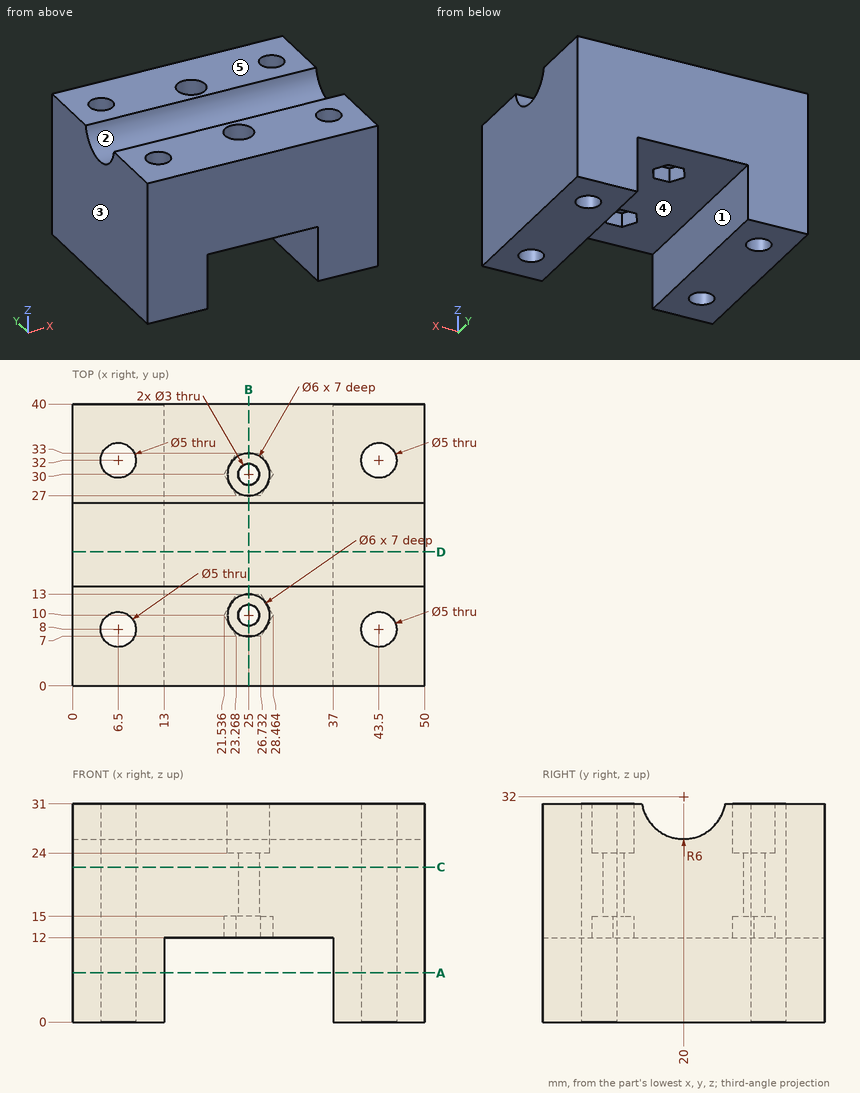
Verification items for this drawing (mm, ordinates from the low corner). A direction names the side the tool comes from. Coordinates: 2 decimals unless noted, no trailing zeros. Write each loop counter-clockwise with the first axis right and the second up, starting at its lowest first coordinate (ties: lowest second). Pieces come first, ordered by that corner, then holes. Notation, with made-up numbers: M 86,30.5 L 123,30.5 A19 cw 123,44.5 Z; hole C 80.25,4.25 d2. An arc over 180 degrees is marked long. Answer as a JSON object with one key per item and string values. Group by question number.
(1) Gauge pin test, flat ends, axial feed: pin 1 (5 mm diameter, centred on x = 30.5, y = 8.5, fed in from -Z); pin 2 (6 mm diameter, centred on x = 31.5, z = 5, fed in from -Y) (1 decimal); pin 3 (5 mm diameter, centred on x = 25, y = 10, fed in from +Z); pin 4 (3.5 mm diameter, centred on x = 25, y = 30, fed in from -Z). Record the tip position at first contact, or that the pin passes through.
(2) Cross-section at B-B, the plane x = 25. State how many separate pieces and enclosed holes the cut face has, and give its area (3 significant figures).
(3) Material ranges on line 1 (Y direction, x = 25, z = 22); line 2 (Y direction, x = 43.5, z = 29); line 3 (X direction, y = 27, z = 9), recorded low to high.
(4) Release check for a two-part mould opening along X. For the marked faces 3, 4 and 5 record: +X half, -X half, draft (parallel to the pull), parting line (faces both ways), or undercut.
(5) Cross-section at C-C, the plane z = 22. Record the cut outline in (x, y), and give its area (3 significant figures).
(6) Cross-section at A-A, the plane z = 7. Record the cut outline in (x, y).
(7) Cross-section at D-D, the plane y = 19. Record the cut outline in (x, z).
(8) Tool access check on the marked faces 1 and 2. Record the directions out of +Z, -Z, +X, -X, +Y, -Y that give a thin tool (end or side, any length) a straight path to the whole face; none if there is none.
Reply:
{
 "1": {"pin 1": "z = 12", "pin 2": "through", "pin 3": "z = 24", "pin 4": "z = 15"},
 "2": {"separate pieces": "3", "enclosed holes": "0", "area": "541 mm²"},
 "3": {"line 1": "0 to 8.5, 11.5 to 28.5, 31.5 to 40", "line 2": "0 to 5.5, 10.5 to 14.8, 25.2 to 29.5, 34.5 to 40", "line 3": "0 to 13, 37 to 50"},
 "4": {"face 3": "-X half", "face 4": "undercut", "face 5": "draft"},
 "5": {"outline": "M 0,0 L 50,0 L 50,40 L 0,40 Z; hole C 6.5,8 d5; hole C 6.5,32 d5; hole C 25,10 d3; hole C 25,30 d3; hole C 43.5,8 d5; hole C 43.5,32 d5", "area": "1,910 mm²"},
 "6": {"outline": "M 0,0 L 13,0 L 13,40 L 0,40 Z; M 37,0 L 50,0 L 50,40 L 37,40 Z; hole C 6.5,8 d5; hole C 6.5,32 d5; hole C 43.5,8 d5; hole C 43.5,32 d5"},
 "7": {"outline": "M 0,0 L 13,0 L 13,12 L 37,12 L 37,0 L 50,0 L 50,26.08 L 0,26.08 Z"},
 "8": {"face 1": "-Z, +Y, -Y", "face 2": "+Z, +X, -X"}
}
